Design review of the part built by this model. Coordinates are the model's own, in mm. A direction names the side the tool comes from. Round coordinates to 2 decimals unless told otherwise and drop trailing zeros. Order: outer loops, then holes, each group sorted by start corner. A loop starts at its lowest first (then second) coordinate and runs counter-clockwise, first axis right, second up.
from build123d import *

# Parameters (mm, degrees)
SKETCH1_W           = 150
SKETCH1_H           = 100
BOSS_EXTRUDE1_DEPTH = 14
SKETCH2_R           = 2.65
CUT_EXTRUDE1_DEPTH  = 15
SKETCH4_R           = 4.6
CUT_EXTRUDE2_DEPTH  = 4
BOSS_EXTRUDE3_START = 15
BOSS_EXTRUDE3_DEPTH = 40
FILLET1_R           = 5


with BuildPart() as part:
    # Sketch1 → Boss-Extrude1 (new body)
    with BuildSketch(Plane(origin=(0, 0, 0), x_dir=(1, 0, 0), z_dir=(0, 1, 0))):
        with Locations((75, 50)):
            Rectangle(SKETCH1_W, SKETCH1_H)
    extrude(amount=BOSS_EXTRUDE1_DEPTH)

    # Sketch2 → Cut-Extrude1 (cut, through all)
    with BuildSketch(Plane(origin=(0, 14, 0), x_dir=(1, 0, 0), z_dir=(0, 1, 0))):
        with Locations((8, 42)):
            Circle(SKETCH2_R)
        with Locations((142, 42)):
            Circle(SKETCH2_R)
        with Locations((75, 42)):
            Circle(SKETCH2_R)
        with Locations((142, 22)):
            Circle(SKETCH2_R)
        with Locations((75, 22)):
            Circle(SKETCH2_R)
        with Locations((8, 22)):
            Circle(SKETCH2_R)
    extrude(amount=-CUT_EXTRUDE1_DEPTH, mode=Mode.SUBTRACT)

    # Sketch4 → Cut-Extrude2 (cut)
    with BuildSketch(Plane(origin=(0, 14, 0), x_dir=(1, 0, 0), z_dir=(0, 1, 0))):
        with Locations((8, 42)):
            Circle(SKETCH4_R)
        with Locations((75, 42)):
            Circle(SKETCH4_R)
        with Locations((142, 42)):
            Circle(SKETCH4_R)
        with Locations((8, 22)):
            Circle(SKETCH4_R)
        with Locations((75, 22)):
            Circle(SKETCH4_R)
        with Locations((142, 22)):
            Circle(SKETCH4_R)
    extrude(amount=-CUT_EXTRUDE2_DEPTH, mode=Mode.SUBTRACT)

    # Sketch6 → Boss-Extrude3 (add)
    with BuildSketch(Plane(origin=(75, 0, 0), x_dir=(0, 0, -1), z_dir=(1, 0, 0)).offset(BOSS_EXTRUDE3_START)):
        with BuildLine():
            Line((0, 14), (100, 14))
            ThreePointArc((100, 14), (50, 22), (0, 14))
        make_face()
    boss_extrude3 = extrude(amount=BOSS_EXTRUDE3_DEPTH)

    # Mirror1: Boss-Extrude3 across plane
    add(boss_extrude3.mirror(Plane(origin=(75, 0, 0), x_dir=(0, 0, 1), z_dir=(1, 0, 0))))

    # Fillet1
    fillet1_edges = [part.edges().sort_by_distance(p)[0] for p in [
        (0, 7, -100),
        (150, 7, -100),
        (150, 7, 0),
        (0, 7, 0),
    ]]
    fillet(fillet1_edges, radius=FILLET1_R)


solid = part.part
1) For faces 1 (the face through (140, 14, -51)), 2 (the face through (60, 17, -49)), 3 (the face through (146.25, 12.03, -40.24)), list the 3-axis set-ups (+Z, -Z, +X, -X, +Y, -Y) from which the entire face can be reached by the end or side of a thin tool; tool diameter is ignored.
Results:
face 1: +Z, -Z, +X, +Y
face 2: +Z, -Z, +Y
face 3: +Y
2) Take a section at B-B on x = 8. Give the boundary of the cut face in (y, z), plus the area to 3 significant figures.
Results:
outline: (0, -100) - (14, -100) - (14, -46.6) - (10, -46.6) - (10, -44.65) - (0, -44.65) - close; (0, -39.35) - (10, -39.35) - (10, -37.4) - (14, -37.4) - (14, -26.6) - (10, -26.6) - (10, -24.65) - (0, -24.65) - close; (0, -19.35) - (10, -19.35) - (10, -17.4) - (14, -17.4) - (14, 0) - (0, 0) - close
area: 1,220 mm2
3) Take a section at D-D on x = 47. Give the boundary of the cut face in (y, z).
Results:
outline: (0, -100) - (14, -100) arc R160.25 ccw to (14, 0) - (0, 0) - close
4) Take a section at A-A on y = 11.5. Give the boundary of the cut face in (x, z).
Results:
outline: (0, -95) arc R5 ccw to (5, -100) - (145, -100) arc R5 ccw to (150, -95) - (150, -5) arc R5 ccw to (145, 0) - (5, 0) arc R5 ccw to (0, -5) - close; hole circle Ø9.2 at (8, -42); hole circle Ø9.2 at (8, -22); hole circle Ø9.2 at (75, -42); hole circle Ø9.2 at (75, -22); hole circle Ø9.2 at (142, -42); hole circle Ø9.2 at (142, -22)
5) To check wall thickness, follow line 1 along X through (y, z) = (5.75, -22); line 2 along Z through (x, y) = (8, 10.8); line 3 along X through (y, z) = (11.25, -22). State the ranges of each line that lie inside material, in increasing order.
Results:
line 1: x = 0 to 5.35, 10.65 to 72.35, 77.65 to 139.35, 144.65 to 150
line 2: z = -100 to -46.6, -37.4 to -26.6, -17.4 to 0
line 3: x = 0 to 3.4, 12.6 to 70.4, 79.6 to 137.4, 146.6 to 150
6) Take a section at C-C on z = -13. Give the boundary of the cut face in (x, y).
Results:
outline: (0, 0) - (150, 0) - (150, 14) - (130, 14) - (130, 17.67) - (90, 17.67) - (90, 14) - (60, 14) - (60, 17.67) - (20, 17.67) - (20, 14) - (0, 14) - close
7) The part is to be moulded in two halves that separate along X. For faces 4 (the face through (0, 7, -49)), 5 (the face through (75, 14, -51)), 6 (the face through (10, 14, -51)), 7 (the face through (144.528, 5.07, -42.796)), say which applies: released by +X, released by -X, zero draft, split by the parting line, or undercut.
Results:
face 4: released by -X
face 5: undercut
face 6: zero draft
face 7: undercut
8) Clearance check with flat-ended pins moving along their axes: P1, Ø6.5, axis at y = 20, z = -46.5, coming from the +X side; P2, Ø7.5, axis at x = 72.5, z = -41.5, coming from the +Y side; P3, Ø9, axis at y = 19.5, z = -39, coming from the -X side; P4, Ø4, axis at x = 8, z = -42, coming from the +Y side. State where each tip first meets the part, or that it passes through.
Results:
P1: stops at x = 130
P2: stops at y = 14
P3: stops at x = 20
P4: passes through
